Autodesk Fusion 360 part; units mm, degrees
sketch "Sketch1" plane through (0, 0, 0) normal (0, 0, 1) x (1, 0, 0)
  line L0 (0, 0) -> (50.8, 0)
  line L1 (50.8, 0) -> (50.8, 50.8)
  line L2 (50.8, 50.8) -> (0, 50.8)
  line L3 (0, 50.8) -> (0, 0)
  dimension "d1" = 50.8
  dimension "d2" = 50.8
extrude "Extrude1" add sketch "Sketch1" along normal blind 31.75
sketch "Sketch2" plane through (50.8, 0, 0) normal (1, 0, 0) x (0, 1, 0)
  line L0 (0, 0) -> (50.8, 0)
  line L1 (50.8, 0) -> (50.8, 31.75)
  line L2 (50.8, 31.75) -> (0, 31.75)
  line L3 (0, 31.75) -> (0, 0)
  line L4 (50.8, 23.368) -> (10.16, 23.368)
  line L5 (10.16, 23.368) -> (10.16, 3.81)
  line L6 (10.16, 3.81) -> (50.8, 3.81)
  line L7 (50.8, 3.81) -> (50.8, 23.368)
  dimension "d5" = 40.64
  dimension "d6" = 19.558
  dimension "d14" = 3.81
extrude "Extrude2" cut sketch "Sketch2" against normal blind 40.64 contours L1 L4 L5 L6 L7
sketch "Sketch3" plane through (0, 0, 31.75) normal (0, 0, 1) x (-1, 0, 0)
  line L0 (0, -50.8) -> (0, 0)
  line L1 (0, 0) -> (-50.8, 0)
  line L2 (-50.8, 0) -> (-50.8, -50.8)
  line L3 (-50.8, -50.8) -> (0, -50.8)
  line L4 (0, 0) -> (-25.4, 0)
  line L5 (-25.4, 0) -> (-25.4, -25.4)
  line L6 (-25.4, -25.4) -> (0, -25.4)
  line L7 (0, -25.4) -> (0, 0)
  dimension "d10" = 25.4
  dimension "d11" = 25.4
extrude "Extrude3" add sketch "Sketch3" along normal blind 152.4 contours L0 L1 L4 L5 L6 L7
fillet "Fillet1" radius 2.54 2 edges at (25.4, 12.7, 31.75) (12.7, 25.4, 31.75)
sketch "Sketch4" plane through (0, 0, 0) normal (0, 0, -1) x (1, 0, 0)
  line L0 (0, 0) -> (0, -50.8)
  line L1 (0, -50.8) -> (50.8, -50.8)
  line L2 (50.8, -50.8) -> (50.8, 0)
  line L3 (50.8, 0) -> (0, 0)
  line L4 (2.54, -2.54) -> (22.86, -2.54)
  line L5 (22.86, -2.54) -> (22.86, -22.86)
  line L6 (22.86, -22.86) -> (2.54, -22.86)
  line L7 (2.54, -22.86) -> (2.54, -2.54)
  dimension "d17" = 2.54
  dimension "d18" = 2.54
  dimension "d19" = 20.32
  dimension "d20" = 20.32
sketch "Sketch5" plane through (0, 0, 0) normal (0, 0, -1) x (1, 0, 0)
  line L0 (5.334, -5.334) -> (20.066, -5.334)
  line L1 (20.066, -5.334) -> (20.066, -20.066)
  line L2 (20.066, -20.066) -> (5.334, -20.066)
  line L3 (5.334, -20.066) -> (5.334, -5.334)
  line L4 (0, -50.8) -> (0, 0)
  line L5 (0, 0) -> (50.8, 0)
  dimension "d37" = 14.732
  dimension "d38" = 14.732
  dimension "d39" = 5.334
  dimension "d40" = 5.334
sketch "Sketch6" plane through (0, 0, 184.15) normal (0, 0, 1) x (-1, 0, 0)
  line L0 (0, -25.4) -> (0, 0)
  line L1 (0, 0) -> (-25.4, 0)
  line L2 (-25.4, 0) -> (-25.4, -25.4)
  line L3 (-25.4, -25.4) -> (0, -25.4)
  line L4 (-2.54, -22.86) -> (-22.86, -22.86)
  line L5 (-22.86, -22.86) -> (-22.86, -2.54)
  line L6 (-22.86, -2.54) -> (-2.54, -2.54)
  line L7 (-2.54, -2.54) -> (-2.54, -22.86)
  line L8 (-5.08, -20.32) -> (-20.32, -20.32)
  line L9 (-20.32, -20.32) -> (-20.32, -5.08)
  line L10 (-20.32, -5.08) -> (-5.08, -5.08)
  line L11 (-5.08, -5.08) -> (-5.08, -20.32)
  dimension "d27" = 2.54
  dimension "d28" = 2.54
  dimension "d29" = 2.54
  dimension "d30" = 20.32
  dimension "d31" = 2.54
  dimension "d32" = 15.24
  dimension "d33" = 15.24
  dimension "d34" = 2.54
extrude "Extrude5" cut sketch "Sketch6" against normal blind 2.54 contours L8 L9 L10 L11
loft "Loft2" cut profiles "Sketch6" section 1 contours L4 L5 L6 L7 section 2 face at (15.24, 15.24, 181.61)
extrude "Extrude6" add sketch "Sketch5" along normal blind 5.08
Source: CAD feature listing. Evaluate the final solid. Frame: model axes, mm. A direction names the side the tool comes from. Give positions to 0.01 mm unless a question says otherwise; leave off trailing zeros. Loops run counter-clockwise (first coordinate to the right, second up) from the corner with the lowest first, then second, coordinate; pieces in that order, holes last. Notation, with made-up numbers: (-19, -24) - (31, -24) arc R23 cw to (31, 0) - close; hole circle Ø10 at (45, 77). An arc over 180 degrees is marked (long way). Use CSV: the item, a comma, the result in double quotes. Start each with the question number.
1. Pin query (flat end, axial travel): pin 1 (6 mm diameter, centred on x = 25.5, z = 12.5, fed in from +Y); pin 2 (1 mm diameter, centred on x = 26.5, y = 38, fed in from +Z); pin 3 (8 mm diameter, centred on x = 6.5, y = 39, fed in from -Z). Return the tip coordinate at first contact, or that it passes through.
2. Section C-C (z = 149.5). Output: boundary loops of the cut face in (x, y).
3. Reachability of faces 4 (the flat face through (5.334, 13, -3)), 5 (the flat face through (31, 31, 31.75)), 6 (the flat face through (13, 25.4, 108)), 7 (the flat face through (13, 13, 181.61)), 8 (the flat face through (20.066, 13, -3)) from +Z, -Z, +X, -X, +Y, -Y: full face, straight path, thin tool, end or side. Return the list, or none.
4. Section A-A (y = 34). Output: boundary loops of the cut face in (x, z).
5. Ray query, L1, parallel to Z at x = 32.5, y = 30; L2, parallel to Z at x = 24.5, y = 14; L3, parallel to Y at x = 16.5, z = 14. Return the intervals inside material, ascending.
6. Draft query along Z for faces 1 (the flat face through (25.4, 13, 108)), 2 (the flat face through (2, 13, 184.15)), 3 (the flat face through (31, 10.16, 14)). Return one class per face: +Z half, -Z half, draft (parallel to the pull), parting line (faces both ways), or undercut.
Response:
1,pin 1,"y = 10.16"
1,pin 2,"z = 31.75"
1,pin 3,"z = 0"
2,outline,"(0, 0) - (25.4, 0) - (25.4, 25.4) - (0, 25.4) - close"
3,face 4,"-Z, -X, +Y, -Y"
3,face 5,"+Z, +X, +Y"
3,face 6,"+Z, +X, -X, +Y"
3,face 7,"+Z"
3,face 8,"-Z, +X, +Y, -Y"
4,outline,"(0, 0) - (50.8, 0) - (50.8, 3.81) - (10.16, 3.81) - (10.16, 23.37) - (50.8, 23.37) - (50.8, 31.75) - (0, 31.75) - close"
5,L1,"0 to 3.81, 23.37 to 31.75"
5,L2,"0 to 3.81, 23.37 to 184.15"
5,L3,"0 to 10.16"
6,face 1,"draft"
6,face 2,"+Z half"
6,face 3,"undercut"
